from build123d import *

# Parameters (mm, degrees)
BOSS_EXTRUDE1_DEPTH = 4
BOSS_EXTRUDE2_DEPTH = 0.3
SKETCH3_R           = 0.35
BOSS_EXTRUDE3_DEPTH = 0.3
FILLET2_R           = 0.15
FILLET3_R           = 0.15
SKETCH4_R           = 3
BOSS_EXTRUDE4_DEPTH = 1.5
SKETCH5_R           = 1
BOSS_EXTRUDE5_DEPTH = 5


with BuildPart() as part:
    # Sketch1 → Boss-Extrude1 (new body)
    with BuildSketch(Plane(origin=(0, 0, 0), x_dir=(1, 0, 0), z_dir=(0, 1, 0))):
        with BuildLine():
            Line((-5, 6), (5, 6))
            ThreePointArc((5, 6), (5.707106781, 5.707106781), (6, 5))
            Line((6, 5), (6, -5))
            ThreePointArc((6, -5), (5.707106781, -5.707106781), (5, -6))
            Line((5, -6), (-5, -6))
            ThreePointArc((-5, -6), (-5.707106781, -5.707106781), (-6, -5))
            Line((-6, -5), (-6, 5))
            ThreePointArc((-6, 5), (-5.707106781, 5.707106781), (-5, 6))
        make_face()
    extrude(amount=BOSS_EXTRUDE1_DEPTH)

    # Sketch2 → Boss-Extrude2 (add)
    with BuildSketch(Plane(origin=(0, 4, 0), x_dir=(1, 0, 0), z_dir=(0, 1, 0))):
        with BuildLine():
            Line((-4.25, 5.25), (4.25, 5.25))
            ThreePointArc((4.25, 5.25), (4.957106781, 4.957106781), (5.25, 4.25))
            Line((5.25, 4.25), (5.25, -4.25))
            ThreePointArc((5.25, -4.25), (4.957106781, -4.957106781), (4.25, -5.25))
            Line((4.25, -5.25), (-4.25, -5.25))
            ThreePointArc((-4.25, -5.25), (-4.957106781, -4.957106781), (-5.25, -4.25))
            Line((-5.25, -4.25), (-5.25, 4.25))
            ThreePointArc((-5.25, 4.25), (-4.957106781, 4.957106781), (-4.25, 5.25))
        make_face()
    extrude(amount=BOSS_EXTRUDE2_DEPTH)

    # Sketch3 → Boss-Extrude3 (add)
    with BuildSketch(Plane(origin=(0, 4.3, 0), x_dir=(1, 0, 0), z_dir=(0, 1, 0))):
        with Locations(Location((4.25, 4.25, 0), (0, 0, 90))):
            Circle(SKETCH3_R)
        with Locations(Location((4.25, -4.25, 0), (0, 0, 90))):
            Circle(SKETCH3_R)
        with Locations(Location((-4.25, -4.25, 0), (0, 0, 90))):
            Circle(SKETCH3_R)
        with Locations(Location((-4.25, 4.25, 0), (0, 0, 90))):
            Circle(SKETCH3_R)
    extrude(amount=BOSS_EXTRUDE3_DEPTH)

    # Fillet2
    fillet2_edges = [part.edges().sort_by_distance(p)[0] for p in [
        (-4.25, 4.6, -3.9),
    ]]
    fillet(fillet2_edges, radius=FILLET2_R)

    # Fillet3
    fillet3_edges = [part.edges().sort_by_distance(p)[0] for p in [
        (4.25, 4.6, -3.9),
        (4.25, 4.6, 4.6),
        (-4.25, 4.6, 4.6),
    ]]
    fillet(fillet3_edges, radius=FILLET3_R)

    # Sketch4 → Boss-Extrude4 (add)
    with BuildSketch(Plane(origin=(0, 4.3, 0), x_dir=(1, 0, 0), z_dir=(0, 1, 0))):
        with Locations(Location((0, 0, 0), (0, 0, 90))):
            Circle(SKETCH4_R)
    extrude(amount=BOSS_EXTRUDE4_DEPTH)

    # Sketch5 → Boss-Extrude5 (add)
    with BuildSketch(Plane.XZ):
        with Locations(Location((2.5, -5.027876242, 0), (0, 0, 256.439715219))):
            Circle(SKETCH5_R)
        with Locations(Location((-2.5, -5.027876242, 0), (0, 0, 90))):
            Circle(SKETCH5_R)
    extrude(amount=BOSS_EXTRUDE5_DEPTH)


solid = part.part
CAD build for the part. Positions are in the model's coordinates, mm. A direction names the side the tool comes from. Give positions to 0.01 mm unless a question says otherwise; leave off trailing zeros. Order: outer loops, then holes, each group sorted by start corner. A loop starts at its lowest first (then second) coordinate and runs counter-clockwise, first axis right, second up. Notation, with made-up numbers: (68, 82) - (122, 82) arc R17 cw to (122, 101) - close; hole circle Ø4 at (38.5, 67). An arc over 180 degrees is marked (long way). Answer in a Markdown table with one row per item.
1. Tool access for faces 1 (the flat face through (2.4, 4.3, 2.3)), 2 (the cylindrical face through (-5.699, 1.972, 5.715)), 3 (the cylindrical face through (1.911, -2.465, -5.836)): list every direction of +Z, -Z, +X, -X, +Y, -Y with a clear straight run to the whole face (end or side of a thin tool).
Data:
| item | result |
|---|---|
| face 1 | +Y |
| face 2 | +Z, -X, +Y, -Y |
| face 3 | -Y |
2. Saw through at B-B, the plane x = 1.25. Give the cut face in (y, z).
Data:
| item | result |
|---|---|
| outline | (0, -6) - (4, -6) - (4, -5.25) - (4.3, -5.25) - (4.3, -2.73) - (5.8, -2.73) - (5.8, 2.73) - (4.3, 2.73) - (4.3, 5.25) - (4, 5.25) - (4, 6) - (0, 6) - close |
3. Saw through at C-C, the plane y = -4.5. Give the cut face in (x, z), plus the area to 3 significant figures.
Data:
| item | result |
|---|---|
| outline | circle Ø2 at (-2.5, -5.03); circle Ø2 at (2.5, -5.03) |
| area | 6.28 mm² |
4. Pull direction X, two halves, no side cores. Call faces 4 (the cylindrical face through (-0.9, 5.04, -2.86)), 5 (the flat face through (0, 2, -6)), 6 (the cylindrical face through (-2.544, -2.465, -6.027)), 7 (the cylindrical face through (-5.715, 1.972, -5.699)): pulls with the +X half, pulls with the -X half, needs draft (parallel to the pull), parting line crosses it, or undercut.
Data:
| item | result |
|---|---|
| face 4 | parting line crosses it |
| face 5 | needs draft |
| face 6 | undercut |
| face 7 | pulls with the -X half |
5. Flat gauge pins, fed straight in: pin 1 (1.5 mm diameter, centred on x = 1.5, y = -1, fed in from -Z); pin 2 (4 mm diameter, centred on x = -4, z = 4.5, fed in from -Y); pin 3 (6 mm diameter, centred on x = -1.5, z = -1.5, fed in from -Y). Where does each tip first touch, or does it go through?
Data:
| item | result |
|---|---|
| pin 1 | stops at z = -6 |
| pin 2 | stops at y = 0 |
| pin 3 | stops at y = -5 |
6. Saw through at A-A, the plane z = -1.25. Give the cut face in (x, y), plus the area to 3 significant figures.
Data:
| item | result |
|---|---|
| outline | (-6, 0) - (6, 0) - (6, 4) - (5.25, 4) - (5.25, 4.3) - (2.73, 4.3) - (2.73, 5.8) - (-2.73, 5.8) - (-2.73, 4.3) - (-5.25, 4.3) - (-5.25, 4) - (-6, 4) - close |
| area | 59.3 mm² |
7. Probe probe 1 along Y at (x, z) = (-0.25, -2.5); probe 2 along Y at (x, z) = (-4.5, -3); probe 3 along Z at (x, y) = (1.25, 2.75). List the from-to ranges inside material, lowest first. Write a range as [from, to].
Data:
| item | result |
|---|---|
| probe 1 | y = [0, 5.8] |
| probe 2 | y = [0, 4.3] |
| probe 3 | z = [-6, 6] |
